Input: part model. Units: mm. Frame: model coordinates. Face numbers are marked on the shaded views. A direction names the side the tool comes from. Coordinates: 2 decimals unless noted, no trailing zeros. Write each loop counter-clockwise with the first axis right and the second up, starting at its lowest first coordinate (ties: lowest second). Pieces come first, ordered by that corner, then holes. Notation, with made-up numbers: M -35,79 L -11,79 A37 cw -11,118 Z; hole C -11.75,-26 d9. An arc over 180 degrees is marked long. Write each question's results on one line, items separated by ' | '. Start each with the question number.
1. Section query D-D, the plane x = 3.5. Output: boundary loops of the cut face in (y, z), and give its area (3 significant figures).
2. Section query C-C, the plane z = 4. Output: boundary loops of the cut face in (x, y).
3. First-contact query: pin 1 (0.6 mm diameter, centred on y = -25.5, z = 1, fed in from -X); pin 2 (2 mm diameter, centred on x = 3.5, z = -4.5, fed in from -Y); pin 3 (4 mm diameter, centred on x = 6.5, z = 1.5, fed in from -Y). Flat tips, straight axial feed; report the tip coordinate or a pass-through.
4. Ray query, probe 1 along X at (y, z) = (-25.5, 1.5); probe 2 along Y at (x, z) = (-6.75, 7); probe 3 along Y at (x, z) = (0.5, 1.5). Return the intervals inside material, ascending.
5. Section query B-B, the plane y = 2. Output: boundary loops of the cut face in (x, z), and give its area (3 significant figures).
6. Set-up query: the marked faces 1 and 2. Return all of +Z, -Z, +X, -X, +Y, -Y with unobstructed straight access to the full face (end or side cutting, diameter ignored); none if empty.
7. Section query A-A, the plane x = 0. Output: boundary loops of the cut face in (y, z).
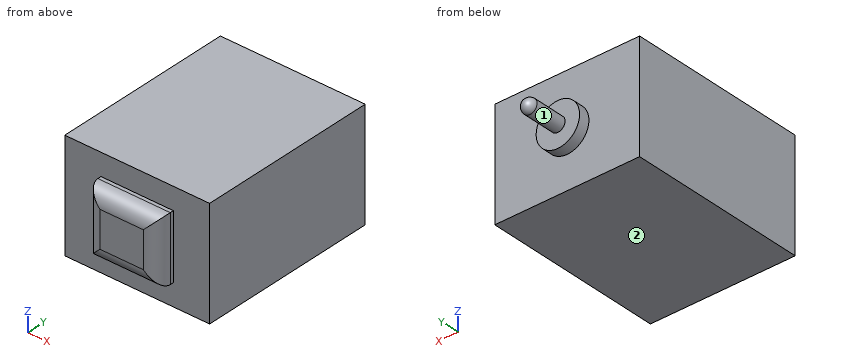
```python
from build123d import *

# Parameters (mm, degrees)
F0_W      = 20
F0_H      = 15.1
F1_DEPTH  = 25
F3_R      = 3
F3_R_2    = 1
F4_DEPTH  = 1.5
F4_FACE_R = 1
F5_DEPTH  = 7
F6_R      = 1
F8_W      = 10
F8_H      = 9
F9_DEPTH  = 2.5
F10_R     = 2


with BuildPart() as f1:
    # F0 (on Front) → F1 (new body)
    with BuildSketch(Plane.XZ):
        Rectangle(F0_W, F0_H)
    extrude(amount=F1_DEPTH)

    # F3 (on offset) → F4 (join)
    with BuildSketch(Plane(origin=(0, 0, 0), x_dir=(1, 0, 0), z_dir=(0, 1, 0))):
        Circle(F3_R)
        Circle(F3_R_2, mode=Mode.SUBTRACT)
    extrude(amount=F4_DEPTH)

    # F4_face (on face) → F5 (join)
    with BuildSketch(Plane(origin=(0, 0, 0), x_dir=(1, 0, 0), z_dir=(0, 1, 0))):
        Circle(F4_FACE_R)
    extrude(amount=F5_DEPTH)

    # F6
    f6_edges = [f1.edges().sort_by_distance(p)[0] for p in [
        (-1, 7, 0),
    ]]
    fillet(f6_edges, radius=F6_R)

    # F8 (on offset) → F9 (join)
    with BuildSketch(Plane.XZ.offset(25)):
        Rectangle(F8_W, F8_H)
    extrude(amount=F9_DEPTH)

    # F10
    f10_edges = [f1.edges().sort_by_distance(p)[0] for p in [
        (0, -27.5, 4.5),
        (5, -27.5, 0),
        (-5, -27.5, 0),
        (0, -27.5, -4.5),
    ]]
    fillet(f10_edges, radius=F10_R)


solid = f1.part
```
Answer:
1) outline: M -27.44,-3 A2 ccw -25.5,-4.5 L -25,-4.5 L -25,-7.55 L 0,-7.55 L 0,7.55 L -25,7.55 L -25,4.5 L -25.5,4.5 A2 ccw -27.44,3 Z | area: 398 mm^2
2) outline: M -10,-25 L -5,-25 L -5,-25.5 A2 ccw -4.5,-26.82 L 4.5,-26.82 A2 ccw 5,-25.5 L 5,-25 L 10,-25 L 10,0 L -10,0 Z
3) pin 1: x = -5 | pin 2: y = -27.23 | pin 3: y = -26.82
4) probe 1: -5 to 5 | probe 2: -25 to 0 | probe 3: -27.5 to 1.5
5) outline: C 0,0 d2 | area: 3.14 mm^2
6) face 1: +Y | face 2: -Z, +X, -X, +Y, -Y
7) outline: M -27.5,-2.5 A2 ccw -25.5,-4.5 L -25,-4.5 L -25,-7.55 L 0,-7.55 L 0,-3 L 1.5,-3 L 1.5,-1 L 6,-1 A1 ccw 6,1 L 1.5,1 L 1.5,3 L 0,3 L 0,7.55 L -25,7.55 L -25,4.5 L -25.5,4.5 A2 ccw -27.5,2.5 Z
